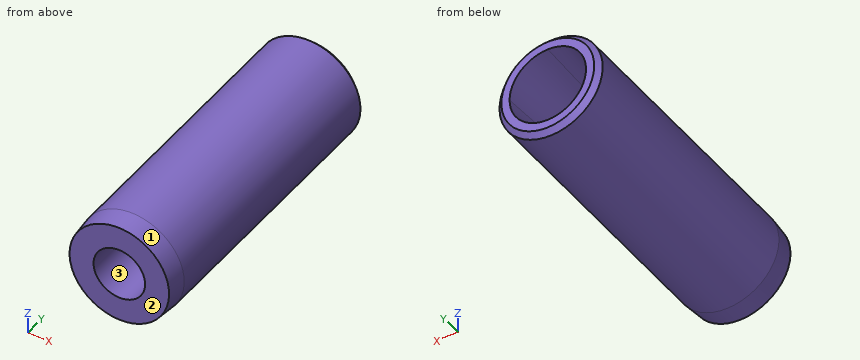
```python
from build123d import *

# Parameters (mm, degrees)
SKETCH1_R           = 5
SKETCH1_R_2         = 2.5
BOSS_EXTRUDE1_DEPTH = 29
CHAMFER1_SIZE       = 2
CHAMFER1_SIZE2      = 0.174977327
CHAMFER2_SIZE       = 0.5


with BuildPart() as part:
    # Sketch1 → Boss-Extrude1 (new body)
    with BuildSketch(Plane(origin=(0, 0, 0), x_dir=(1, 0, 0), z_dir=(0, 1, 0))):
        with Locations(Location((0, 0, 0), (0, 0, 90))):
            Circle(SKETCH1_R)
        with Locations(Location((0, 0, 0), (0, 0, 90))):
            Circle(SKETCH1_R_2, mode=Mode.SUBTRACT)
    extrude(amount=BOSS_EXTRUDE1_DEPTH)

    # Cut-Sweep1: sweep along a curve in space
    with BuildLine() as cut_sweep1_path:
        ThreePointArc((0, 29, 2.5), (1.767766953, 29, 1.767766953), (2.5, 29, 0))
        ThreePointArc((2.5, 29, 0), (1.767766953, 29, -1.767766953), (0, 29, -2.5))
        ThreePointArc((0, 29, -2.5), (-1.767766953, 29, -1.767766953), (-2.5, 29, 0))
        ThreePointArc((-2.5, 29, 0), (-1.767766953, 29, 1.767766953), (0, 29, 2.5))
    # Sketch2 → Cut-Sweep1 (sweep, cut)
    with BuildSketch(Plane.XY):
        Polygon((2.5, 6), (3.705378924, 29), (2.5, 29), align=None)
    sweep(path=cut_sweep1_path.line, mode=Mode.SUBTRACT)

    # Chamfer1
    chamfer1_edges = [part.edges().sort_by_distance(p)[0] for p in [
        (0, 0, 5),
    ]]
    chamfer1_side = [part.faces().sort_by_distance(p)[0] for p in [
        (0, 14.5, 5),
    ]]
    chamfer(chamfer1_edges, length=CHAMFER1_SIZE, length2=CHAMFER1_SIZE2, reference=chamfer1_side[0])

    # Chamfer2
    chamfer2_edges = [part.edges().sort_by_distance(p)[0] for p in [
        (0, 29, 5),
    ]]
    chamfer(chamfer2_edges, length=CHAMFER2_SIZE)


solid = part.part
```
CAD build for the part. Positions are in the model's coordinates, mm. Face numbers are marked on the shaded views. Coordinates: 2 decimals unless noted, no trailing zeros. Write each loop counter-clockwise with the first axis right and the second up, starting at its lowest first coordinate (ties: lowest second). Pieces come first, ordered by that corner, then holes.
(1) Flat gauge pins, fed straight in: pin 1 (1 mm diameter, centred on x = 2, y = 19.5, fed in from +Z); pin 2 (6 mm diameter, centred on y = 19, z = 0.5, fed in from +X); pin 3 (3 mm diameter, centred on y = 19.5, z = -4, fed in from +X); pin 4 (3 mm diameter, centred on x = -2.5, y = 19.5, fed in from +Z). Where does each tip first touch, or does it go through?
(2) Cut at C-C, the plane y = 25.5. List the corners of the cut face in (x, z), and give its area (3 significant figures).
(3) Drill centre lines: probe 1 along X at (y, z) = (3.9, 0); probe 2 along X at (y, z) = (1.75, 0.5); probe 3 along Z at (x, y) = (1.5, 4.75). Where is each one in solid material? Low to high.
(4) Cut at B-B, the plane y = 17. List the corners of the cut face in (x, z).
(5) Two-plate mould, pull along X, no slides. Class the marked faces 1, 2 and 3: +X half, -X half, draft (parallel to the pull), parting line (faces both ways), or undercut.
(6) Cut at A-A, the plane y = 2.5. List the corners of the cut face in (x, z), and give its area (3 significant figures).
Geometry says:
1. pin 1: stops at z = 4.77
1. pin 2: stops at x = 5
1. pin 3: stops at x = 4.33
1. pin 4: stops at z = 4.9
2. outline: circle Ø10 at (0, 0); hole circle Ø7.04 at (0, 0)
2. area: 39.6 mm2
3. probe 1: x = -5 to -2.5, 2.5 to 5
3. probe 2: x = -4.95 to -2.45, 2.45 to 4.95
3. probe 3: z = -4.77 to -2, 2 to 4.77
4. outline: circle Ø10 at (0, 0); hole circle Ø6.15 at (0, 0)
5. face 1: parting line
5. face 2: draft
5. face 3: undercut
6. outline: circle Ø10 at (0, 0); hole circle Ø5 at (0, 0)
6. area: 58.9 mm2
